Can you work these out from the model? Positions are in its coordinate system, mm. Face numbers are marked on the shaded views. A direction names the side the tool comes from. Coordinates: 2 decimals unless noted, no trailing zeros. Order: outer loops, then holes, each group sorted by start corner. A loop starts at its lowest first (then second) coordinate and runs counter-clockwise, first axis right, second up. Notation, with made-up numbers: (-26, 62.25) - (31, 62.25) arc R36 cw to (31, 99.25) - close; hole circle Ø1 at (39.25, -32.5). An arc over 180 degrees is marked (long way). Return JSON: item names as keys, results as strings. Group by question number.
1) Imagine slicing it at B-B (z = 6.35). Write out the boundary of the cut face in (x, y) (3 decimals).
2) Imagine slicing it at D-D (z = 10.5). Write out the boundary of the cut face in (x, y), and give its area (3 significant figures).
3) If we mould it in two halves opening along X, with no side actions, what happens to the marked faces 1, 2, 3 and 4? For each: pulls with the +X half, pulls with the -X half, needs draft (parallel to the pull), parting line crosses it, or undercut.
4) Which directions (+Z, -Z, +X, -X, +Y, -Y) give clear straight access to the entire face, cutting with the end or side of a thin tool? Please do the marked faces 5, 6, 7 and 8.
5) Imagine slicing it at A-A (x = 17.78). Write out the boundary of the cut face in (y, z) (3 decimals), and give its area (3 significant figures).
6) If I drill on line 1 along X through (y, z) = (10.1, 6.35) (3 decimals); line 2 along Y through (x, z) = (-1.45, 6.35) (3 decimals); line 3 along X through (y, z) = (-4, 9.25), over which ranges is the centre line in solid material (lowest first)?
7) Imagine slicing it at C-C (y = -10.16). Write out the boundary of the cut face in (x, z) (3 decimals), and give its area (3 significant figures).
8) For pin 1 Ø2 at (x, z) = (14.5, 6) entering from -Y; pin 2 Ø4 at (x, z) = (19, 4) entering from +Y; pin 3 Ø4 at (y, z) = (-6, 5.5) entering from +X, each with a flat end and sliding along its axis, tell me the tip position at first contact or that it passes through.
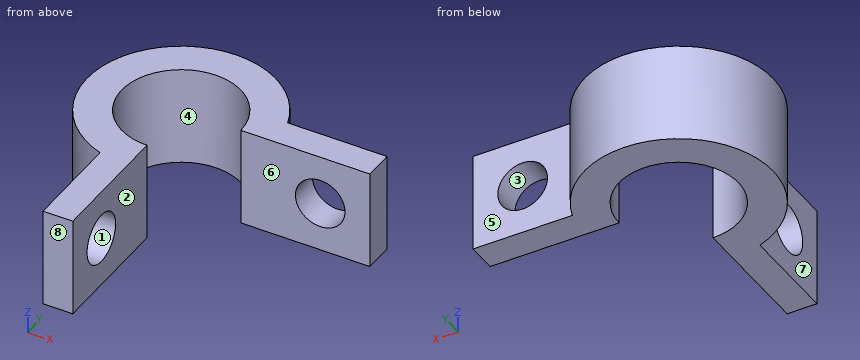
```python
from build123d import *

# Parameters (mm, degrees)
BOSS_EXTRUDE1_DEPTH = 12.7
SKETCH2_R           = 3.175
CUT_EXTRUDE1_DEPTH  = 40.040882418
SKETCH3_R           = 3.175
CUT_EXTRUDE2_DEPTH  = 37.452362817


with BuildPart() as part:
    # Sketch1 → Boss-Extrude1 (new body)
    with BuildSketch(Plane.XY):
        with BuildLine():
            Line((-3.81, -3.81), (-3.81, -16.51))
            Line((-3.81, -16.51), (0, -16.51))
            Line((0, -16.51), (0, 0))
            ThreePointArc((0, 0), (-5.388153673, 13.008153673), (7.62, 7.62))
            Line((7.62, 7.62), (24.13, 7.62))
            Line((24.13, 7.62), (24.13, 11.43))
            Line((24.13, 11.43), (11.43, 11.43))
            ThreePointArc((11.43, 11.43), (-8.519418994, 16.139418994), (-3.81, -3.81))
        make_face()
    extrude(amount=BOSS_EXTRUDE1_DEPTH)

    # Sketch2 → Cut-Extrude1 (cut, through all)
    with BuildSketch(Plane(origin=(0, 11.43, 0), x_dir=(1, 0, 0), z_dir=(0, 1, 0))):
        with Locations(Location((17.78, -6.35, 0), (0, 0, 270))):
            Circle(SKETCH2_R)
    extrude(amount=-CUT_EXTRUDE1_DEPTH, mode=Mode.SUBTRACT)

    # Sketch3 → Cut-Extrude2 (cut, through all)
    with BuildSketch(Plane.ZY.offset(3.81)):
        with Locations((6.35, -10.16)):
            Circle(SKETCH3_R)
    extrude(amount=-CUT_EXTRUDE2_DEPTH, mode=Mode.SUBTRACT)


solid = part.part
```
Calculated:
{
 "1": {"outline": "(-3.81, -16.51) - (0, -16.51) - (0, -13.335) - (-3.81, -13.335) - close; (-3.81, -6.985) - (0, -6.985) - (0, 0) arc R7.62 cw (long way) to (7.62, 7.62) - (14.605, 7.62) - (14.605, 11.43) - (11.43, 11.43) arc R12.048 ccw (long way) to (-3.81, -3.81) - close; (20.955, 7.62) - (24.13, 7.62) - (24.13, 11.43) - (20.955, 11.43) - close"},
 "2": {"outline": "(-3.81, -16.51) - (0, -16.51) - (0, 0) arc R7.62 cw (long way) to (7.62, 7.62) - (24.13, 7.62) - (24.13, 11.43) - (11.43, 11.43) arc R12.05 ccw (long way) to (-3.81, -3.81) - close", "area": "299 mm2"},
 "3": {"face 1": "needs draft", "face 2": "pulls with the +X half", "face 3": "undercut", "face 4": "undercut"},
 "4": {"face 5": "+Z, -Z, +X, +Y", "face 6": "+Z, -Z, +X, -Y", "face 7": "+Z, -Z, -X, -Y", "face 8": "+Z, -Z, +X, -X, -Y"},
 "5": {"outline": "(7.62, 0) - (11.43, 0) - (11.43, 3.175) - (7.62, 3.175) - close; (7.62, 9.525) - (11.43, 9.525) - (11.43, 12.7) - (7.62, 12.7) - close", "area": "24.2 mm2"},
 "6": {"line 1": "-11.79 to -7.205, 7.205 to 14.605, 20.955 to 24.13", "line 2": "-16.51 to -13.335, -6.985 to 0.139, 15.101 to 19.581", "line 3": "-3.81 to 0"},
 "7": {"outline": "(-3.81, 0) - (0, 0) - (0, 3.175) - (-3.81, 3.175) - close; (-3.81, 9.525) - (0, 9.525) - (0, 12.7) - (-3.81, 12.7) - close", "area": "24.2 mm2"},
 "8": {"pin 1": "y = 7.62", "pin 2": "y = 11.43", "pin 3": "x = 0"}
}
